```python
from build123d import *

# Parameters (mm, degrees)
BOSS_EXTRUDE1_DEPTH = 1.524
SKETCH2_R           = 3.175
CUT_EXTRUDE1_DEPTH  = 62.84577276
SKETCH3_W           = 31.75
SKETCH3_H           = 1.5875
BOSS_EXTRUDE2_DEPTH = 14.224
FILLET1_R           = 1.5875
SKETCH4_R           = 2.54
CUT_EXTRUDE2_DEPTH  = 64.801070024


with BuildPart() as part:
    # Sketch1 → Boss-Extrude1 (new body)
    with BuildSketch(Plane.XY):
        with BuildLine():
            Line((-24.150754652, 16.594156681), (-15.875, 0))
            Line((-15.875, 0), (15.875, 0))
            Line((15.875, 0), (24.150754652, 16.594156681))
            ThreePointArc((24.150754652, 16.594156681), (0, 55.626), (-24.150754652, 16.594156681))
        make_face()
    extrude(amount=BOSS_EXTRUDE1_DEPTH)

    # Sketch2 → Cut-Extrude1 (cut, through all)
    with BuildSketch(Plane.XY.offset(1.524)):
        with Locations((0, 28.6385)):
            Circle(SKETCH2_R)
    extrude(amount=-CUT_EXTRUDE1_DEPTH, mode=Mode.SUBTRACT)

    # Sketch3 → Boss-Extrude2 (add)
    with BuildSketch(Plane.XY.offset(1.524)):
        with Locations((0, 0.79375)):
            Rectangle(SKETCH3_W, SKETCH3_H)
    extrude(amount=BOSS_EXTRUDE2_DEPTH)

    # Fillet1
    # the kernel refuses this fillet: 1.5875 mm, written as the material it adds along each edge
    with BuildSketch(Plane(origin=(15.875, 1.5875, 1.524), x_dir=(0, 1, 0), z_dir=(-1, 0, 0))) as fillet1_piece_1:
        with BuildLine():
            CenterArc((FILLET1_R, -FILLET1_R), FILLET1_R, 90, 90)
            Line((0, -FILLET1_R), (0, 0))
            Line((0, 0), (FILLET1_R, 0))
        make_face()
    extrude(amount=31.75)
    # the kernel refuses this fillet: 1.5875 mm, written as the material it takes off along each edge
    with BuildSketch(Plane(origin=(-15.875, 5.55625, 15.748), x_dir=(1, 0, 0), z_dir=(0, -1, 0))) as fillet1_2_piece_1:
        with BuildLine():
            CenterArc((FILLET1_R, -FILLET1_R), FILLET1_R, 90, 90)
            Line((0, -FILLET1_R), (0, 0))
            Line((0, 0), (FILLET1_R, 0))
        make_face()
    extrude(amount=9.525, mode=Mode.SUBTRACT)
    with BuildSketch(Plane(origin=(15.875, -3.96875, 15.748), x_dir=(0, 0, -1), z_dir=(0, 1, 0))) as fillet1_2_piece_2:
        with BuildLine():
            CenterArc((FILLET1_R, FILLET1_R), FILLET1_R, 180, 90)
            Line((0, FILLET1_R), (0, 0))
            Line((0, 0), (FILLET1_R, 0))
        make_face()
    extrude(amount=9.525, mode=Mode.SUBTRACT)
    with BuildSketch(Plane(origin=(-19.84375, 0, 0), x_dir=(0, 1, 0), z_dir=(1, 0, 0))) as fillet1_2_piece_3:
        with BuildLine():
            CenterArc((FILLET1_R, FILLET1_R), FILLET1_R, 180, 90)
            Line((0, FILLET1_R), (0, 0))
            Line((0, 0), (FILLET1_R, 0))
        make_face()
    extrude(amount=39.6875, mode=Mode.SUBTRACT)

    # Sketch4 → Cut-Extrude2 (cut, through all)
    with BuildSketch(Plane.XZ):
        with Locations(Location((7.62, 9.398, 0), (0, 0, 270))):
            Circle(SKETCH4_R)
        with Locations(Location((-7.62, 9.398, 0), (0, 0, 270))):
            Circle(SKETCH4_R)
    extrude(amount=-CUT_EXTRUDE2_DEPTH, mode=Mode.SUBTRACT)


solid = part.part
```
Source: CAD feature listing. Evaluate the final solid. Frame: model axes, mm. A direction names the side the tool comes from. Round coordinates to 2 decimals unless told otherwise and drop trailing zeros. Loops run counter-clockwise (first coordinate to the right, second up) from the corner with the lowest first, then second, coordinate; pieces in that order, holes last. Notation, with made-up numbers: M -18.5,66.5 L 15.5,66.5 A23 ccw 15.5,93.5 Z; hole C 29,59.5 d2. An arc over 180 degrees is marked long. Use a Markdown table: item, result. Add a question column.
1. Cut plane A-A, the plane x = 0. Output: boundary loops of the cut face in (y, z) (1 decimal), and give its area (3 significant figures).
2. Contact query for flat-ended pins moving along their axis: pin 1 (4.5 mm diameter, centred on x = 7.62, z = 9.398, fed in from -Y); pin 2 (5 mm diameter, centred on x = 21.5, z = 2, fed in from +Y); pin 3 (4 mm diameter, centred on x = 0, z = 12, fed in from +Y); pin 4 (1.6 mm diameter, centred on y = 1.5, z = 6.5, fed in from -X) (3 decimals). Output: stop coordinate, or through.
3. Cut plane C-C, the plane x = 11. Output: boundary loops of the cut face in (y, z) (1 decimal), and give its area (3 significant figures).
4. Cut plane D-D, the plane x = -7.62. Output: boundary loops of the cut face in (y, z) (1 decimal), and give its area (3 significant figures).
5. Cut plane B-B, the plane y = 30. Output: boundary loops of the cut face in (x, z).
6. Ray query, line 1 along Z through (x, y) = (7, 1); line 2 along Z through (x, y) = (-11, 16); line 3 along Y through (x, z) = (5, 10.5). Return the intervals inside material, ascending. Write a range as [from, to].
7. Pull-direction query (X, two-part tool) for faces 1 (the cylindrical face through (-0.69, 25.54, 0.77)), 2 (the cylindrical face through (0.768, 55.615, 0.751)), 3 (the flat face through (-20.07, 8.41, 0.75)); classes: +X half, -X half, draft (parallel to the pull), parting line (faces both ways), or undercut.
8. Set-up query: faces 4 (the flat face through (0, 1, 15.748)), 5 (the flat face through (15.875, 1, 8)), 6 (the cylindrical face through (6.07, 0.78, 11.41)), 7 (the flat face through (0, 1.588, 9)), 8 (the flat face through (-15.875, 1, 8)). Return all of +Z, -Z, +X, -X, +Y, -Y with unobstructed straight access to the full face (end or side cutting, diameter ignored); none if empty.
Solution:
| question | item | result |
|---|---|---|
| 1 | outline | M 0,1.6 A1.6 ccw 1.6,0 L 25.5,0 L 25.5,1.5 L 3.2,1.5 A1.6 cw 1.6,3.1 L 1.6,15.7 L 0,15.7 Z; M 31.8,0 L 55.6,0 L 55.6,1.5 L 31.8,1.5 Z |
| 1 | area | 97.7 mm2 |
| 2 | pin 1 | passes through |
| 2 | pin 2 | stops at y = 47.76 |
| 2 | pin 3 | stops at y = 1.59 |
| 2 | pin 4 | stops at x = -15.875 |
| 3 | outline | M 0,1.6 A1.6 ccw 1.6,0 L 53.3,0 L 53.3,1.5 L 3.2,1.5 A1.6 cw 1.6,3.1 L 1.6,15.7 L 0,15.7 Z |
| 3 | area | 104 mm2 |
| 4 | outline | M 0,1.6 A1.6 ccw 1.6,0 L 54.5,0 L 54.5,1.5 L 3.2,1.5 A1.6 cw 1.6,3.1 L 1.6,6.9 L 0,6.9 Z; M 0,11.9 L 1.6,11.9 L 1.6,15.7 L 0,15.7 Z |
| 4 | area | 97.6 mm2 |
| 5 | outline | M -26.95,0 L -2.87,0 L -2.87,1.52 L -26.95,1.52 Z; M 2.87,0 L 26.95,0 L 26.95,1.52 L 2.87,1.52 Z |
| 6 | line 1 | z = [0.11, 6.93], [11.86, 15.75] |
| 6 | line 2 | z = [0, 1.52] |
| 6 | line 3 | y = [0, 1.59] |
| 7 | face 1 | undercut |
| 7 | face 2 | parting line |
| 7 | face 3 | -X half |
| 8 | face 4 | +Z, +X, -X, +Y, -Y |
| 8 | face 5 | +Z, +X, +Y, -Y |
| 8 | face 6 | +Y, -Y |
| 8 | face 7 | +Z, +X, -X, +Y |
| 8 | face 8 | +Z, -X, +Y, -Y |
